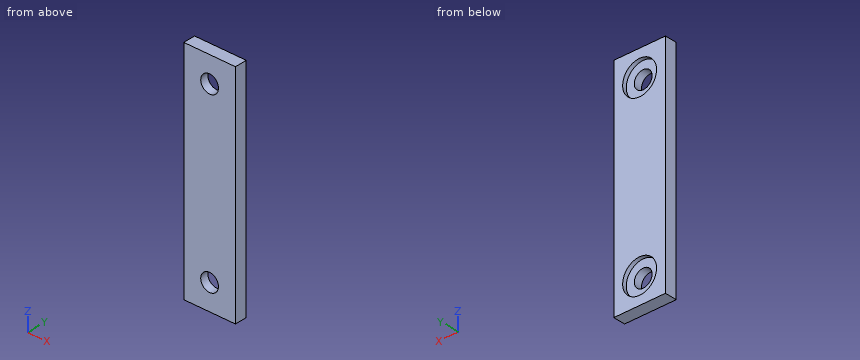
from build123d import *

# Parameters (mm, degrees)
SKETCH_1_W          = 6.4
SKETCH_1_H          = 28
EXTRUDE_1_DEPTH     = 1.5
SKETCH_2_R          = 1.1
CUT_EXTRUDE_1_DEPTH = 15.439182802
SKETCH_3_R          = 2.1
CUT_EXTRUDE_2_DEPTH = 0.5


with BuildPart() as part:
    # Эскиз1 → Бобышка-Вытянуть1 (new body)
    with BuildSketch(Plane(origin=(0, 0, 0), x_dir=(1, 0, 0), z_dir=(0, 1, 0))):
        Rectangle(SKETCH_1_W, SKETCH_1_H)
    extrude(amount=EXTRUDE_1_DEPTH)

    # Эскиз2 → Вырез-Вытянуть1 (cut, through all)
    with BuildSketch(Plane(origin=(0, 1.5, 0), x_dir=(1, 0, 0), z_dir=(0, 1, 0))):
        with Locations(Location((0, 10.8, 0), (0, 0, 270))):
            Circle(SKETCH_2_R)
        with Locations(Location((0, -10.8, 0), (0, 0, 90))):
            Circle(SKETCH_2_R)
    extrude(amount=-CUT_EXTRUDE_1_DEPTH, mode=Mode.SUBTRACT)

    # Эскиз3 → Вырез-Вытянуть2 (cut)
    with BuildSketch(Plane(origin=(0, 1.5, 0), x_dir=(1, 0, 0), z_dir=(0, 1, 0))):
        with Locations(Location((0, 10.8, 0), (0, 0, 270))):
            Circle(SKETCH_3_R)
        with Locations(Location((0, -10.8, 0), (0, 0, 270))):
            Circle(SKETCH_3_R)
    extrude(amount=-CUT_EXTRUDE_2_DEPTH, mode=Mode.SUBTRACT)


solid = part.part
Source: CAD feature listing. Evaluate the final solid. Frame: model axes, mm. Give positions to 0.01 mm unless a question says otherwise; leave off trailing zeros. Write each loop counter-clockwise with the first axis right and the second up, starting at its lowest first coordinate (ties: lowest second). Pieces come first, ordered by that corner, then holes. Notation, with made-up numbers: (8.5, 14.5) -> (44.5, 14.5) arc R17 ccw to (44.5, 44.5) -> close; hole circle Ø10 at (15.25, 88.5). An arc over 180 degrees is marked (long way). Write item = value, one per line.
Q1. Cut plane B-B on y = 0.7. Return loops of the section in (x, z), then the cut area to 3 significant figures.
Here are the results:
outline = (-3.2, -14) -> (3.2, -14) -> (3.2, 14) -> (-3.2, 14) -> close; hole circle Ø2.2 at (0, -10.8); hole circle Ø2.2 at (0, 10.8)
area = 172 mm²
Q2. First-contact query: pin 1 (3.5 mm diameter, centred on x = 0, z = 10.8, fed in from +Y); pin 2 (1.8 mm diameter, centred on x = 0, z = -10.8, fed in from -Y). Flat tips, straight axial feed; report the tip coordinate or a pass-through.
Here are the results:
pin_1 = 1
pin_2 = through
Q3. Cut plane A-A on x = 0. Return loops of the section in (y, z).
Here are the results:
outline = (0, -14) -> (1.5, -14) -> (1.5, -12.9) -> (1, -12.9) -> (1, -11.9) -> (0, -11.9) -> close; (0, -9.7) -> (1, -9.7) -> (1, -8.7) -> (1.5, -8.7) -> (1.5, 8.7) -> (1, 8.7) -> (1, 9.7) -> (0, 9.7) -> close; (0, 11.9) -> (1, 11.9) -> (1, 12.9) -> (1.5, 12.9) -> (1.5, 14) -> (0, 14) -> close
Q4. Cut plane C-C on z = 10.8. Return loops of the section in (x, y), then the cut area to 3 significant figures.
Here are the results:
outline = (-3.2, 0) -> (-1.1, 0) -> (-1.1, 1) -> (-2.1, 1) -> (-2.1, 1.5) -> (-3.2, 1.5) -> close; (1.1, 0) -> (3.2, 0) -> (3.2, 1.5) -> (2.1, 1.5) -> (2.1, 1) -> (1.1, 1) -> close
area = 5.30 mm²
Q5. Cut plane D-D on x = -1.5. Return loops of the section in (y, z), then the cut area to 3 significant figures.
Here are the results:
outline = (0, -14) -> (1.5, -14) -> (1.5, -12.27) -> (1, -12.27) -> (1, -9.33) -> (1.5, -9.33) -> (1.5, 9.33) -> (1, 9.33) -> (1, 12.27) -> (1.5, 12.27) -> (1.5, 14) -> (0, 14) -> close
area = 39.1 mm²
Q6. Line query: line 1 (X direction, y = 0.2, z = -10.8); line 2 (X direction, y = 1.2, z = -10.8); line 3 (Z direction, x = 1.25, y = 1.35). Output: solid intervals per line, ascending. Write a range as from..to.
Here are the results:
line_1 = -3.2..-1.1, 1.1..3.2
line_2 = -3.2..-2.1, 2.1..3.2
line_3 = -14..-12.49, -9.11..9.11, 12.49..14
